Check sheet for the drawn part. Datum: minimum x, y, z corner. Units: mm. Give positions to 0.01 mm unless a question says otherwise; leave off trailing zeros. Order: outer loops, then holes, each group sorted by start corner. A loop starts at its lowest first (then second) coordinate and runs counter-clockwise, first axis right, second up.
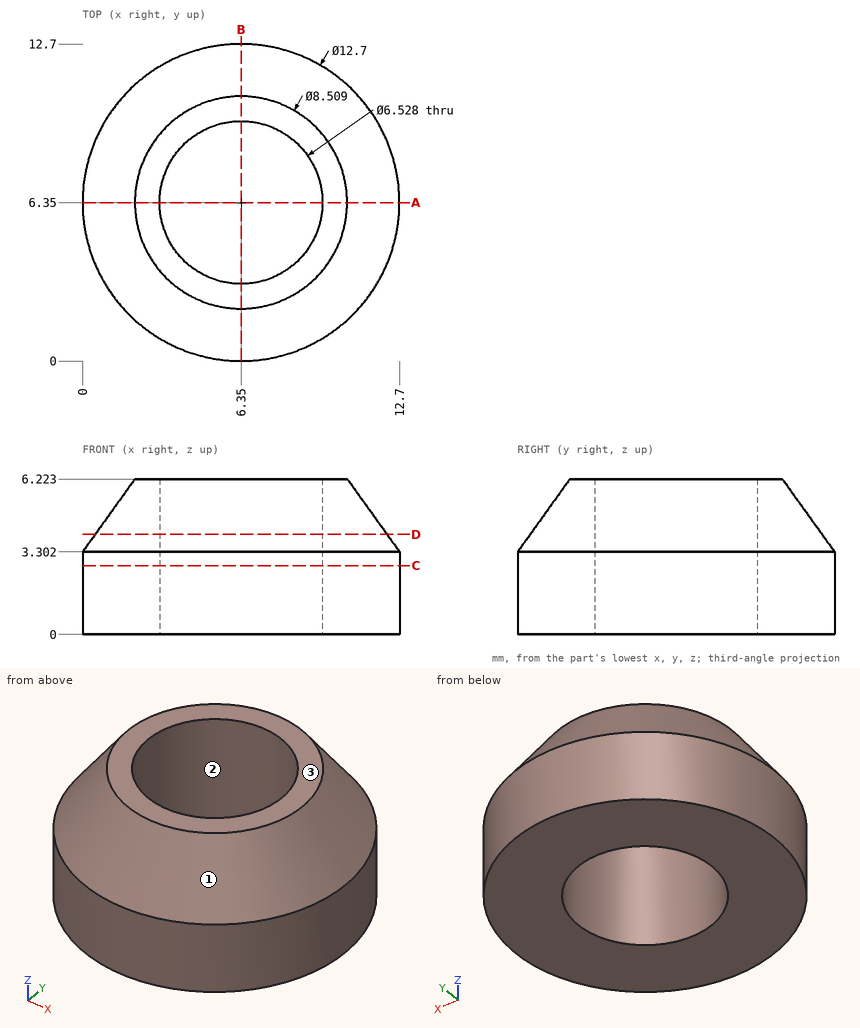
Item 1: Scan lines: L1, parallel to Y at x = 6.35, z = 3.25; L2, parallel to Y at x = 6.35, z = 3.5. Record each from-to range of solid material in increasing order.
Reported:
L1: y = 0 to 3.09, 9.61 to 12.7
L2: y = 0.14 to 3.09, 9.61 to 12.56
Item 2: Gauge pin test, flat ends, axial feed: pin 1 (1 mm diameter, centred on x = 4.5, z = 2.5, fed in from +Y) (1 decimal); pin 2 (2 mm diameter, centred on x = 8, z = 0.5, fed in from +Y). Record the tip position at first contact, or that the pin passes through.
Reported:
pin 1: stops at y = 12.6
pin 2: stops at y = 12.67
Item 3: Draft check along Y on the marked faces 1, 2 and 3. Enter one of: released by +Y, released by -Y, zero draft, split by the parting line, or undercut.
Reported:
face 1: split by the parting line
face 2: undercut
face 3: zero draft
Item 4: Sectioned sample at C-C (z = 2.75). Enter the section's corners in (x, y).
Reported:
outline: circle Ø12.7 at (6.35, 6.35); hole circle Ø6.53 at (6.35, 6.35)
Item 5: Sectioned sample at A-A (y = 6.35). Enter the section's corners in (x, z).
Reported:
outline: (0, 0) - (3.09, 0) - (3.09, 6.22) - (2.1, 6.22) - (0, 3.3) - close; (9.61, 0) - (12.7, 0) - (12.7, 3.3) - (10.6, 6.22) - (9.61, 6.22) - close
Item 6: Sectioned sample at D-D (z = 4). Enter the section's corners in (x, y), and give its area (3 significant figures).
Reported:
outline: circle Ø11.7 at (6.35, 6.35); hole circle Ø6.53 at (6.35, 6.35)
area: 74.0 mm2
